Work out the finished part from the listing and answer in its coordinate system (mm). A direction names the side the tool comes from. Give positions to 0.01 mm unless a question says otherwise; leave off trailing zeros. Loops run counter-clockwise (first coordinate to the right, second up) from the corner with the lowest first, then second, coordinate; pieces in that order, holes last.
```python
from build123d import *

# Parameters (mm, degrees)
F0_R     = 119
F1_DEPTH = 20


with BuildPart() as f1:
    # F0 (on Top) → F1 (new body)
    with BuildSketch(Plane.XY):
        Circle(F0_R)
        with BuildLine():
            Line((-14, -77.585713), (-14, -65.009615))
            ThreePointArc((-14, -65.009615), (-66.126354, 7.039553), (0, 66.5))
            ThreePointArc((0, 66.5), (47.022601, 47.022601), (66.5, 0))
            ThreePointArc((66.5, 0), (51.736109, -41.780677), (14, -65.009615))
            Line((14, -65.009615), (14, -77.585713))
            Line((14, -77.585713), (-14, -77.585713))
        make_face(mode=Mode.SUBTRACT)
    extrude(amount=F1_DEPTH)


solid = f1.part
```
Q1. Which of the six approach directions +Z, -Z, +X, -X, +Y, -Y give full straight-line access (tool end or side, diameter ignored) to faces 1 (the face through (-14, -71, 10)), 2 (the face through (51, -51, 0))?
Q2. Section A-A on z = 11.75 is taken. Give the vertices of the cut face in (x, y).
Q3. Determine the mould class of faces 3 (the face through (51, -51, 20)), 4 (the face through (0, -77.586, 10)), 5 (the face through (14, -71, 10)), 6 (the face through (63.974, 100.341, 9.86)) for opening direction Y: +Y half, -Y half, draft (parallel to the pull), parting line (faces both ways), or undercut.
Q4. Section B-B on y = -11 is taken. Give the vertices of the cut face in (x, z).
Q5. Section D-D on y = -92 is taken. Give the vertices of the cut face in (x, z).
Q6. Consider line 1 along X through (y, z) = (1, 17.5); line 2 along Y through (x, z) = (-19, 1.25); line 3 along X through (y, z) = (-9, 12). Determine where each line is inside the solid, lowest interval first.
Q7. Given pin 1 (3 mm diameter, centred on x = -69.5, y = 9.5, fed in from -Z); pin 2 (4 mm diameter, centred on y = -68.5, z = 5.5, fed in from -X); pin 3 (1 mm diameter, centred on y = 13.5, z = 11, fed in from -X); pin 4 (4 mm diameter, centred on y = -36, z = 14, fed in from +X), each flat-ended and moving along its own axis, determine where each tip first touches the part or whether it passes through.
Q8. Section C-C on y = 17 is taken. Give the vertices of the cut face in (x, z).
Check result:
1. face 1: +Z, -Z
1. face 2: -Z, +X, -X, +Y, -Y
2. outline: circle Ø238 at (0, 0); hole (-14, -77.59) - (14, -77.59) - (14, -65.01) arc R66.5 ccw to (66.5, 0) arc R66.5 ccw (long way) to (-14, -65.01) - close
3. face 3: draft
3. face 4: undercut
3. face 5: undercut
3. face 6: parting line
4. outline: (-118.49, 0) - (-65.58, 0) - (-65.58, 20) - (-118.49, 20) - close; (65.58, 0) - (118.49, 0) - (118.49, 20) - (65.58, 20) - close
5. outline: (-75.48, 0) - (75.48, 0) - (75.48, 20) - (-75.48, 20) - close
6. line 1: x = -119 to -66.49, 66.49 to 119
6. line 2: y = -117.47 to -63.73, 63.73 to 117.47
6. line 3: x = -118.66 to -65.89, 65.89 to 118.66
7. pin 1: stops at z = 0
7. pin 2: stops at x = -98.69
7. pin 3: stops at x = -118.29
7. pin 4: stops at x = 114.04
8. outline: (-117.78, 0) - (-64.29, 0) - (-64.29, 20) - (-117.78, 20) - close; (64.29, 0) - (117.78, 0) - (117.78, 20) - (64.29, 20) - close
